```python
from build123d import *

# Parameters (mm, degrees)
SKETCH1_R              = 9.525
BOSS_EXTRUDE1_DEPTH    = 3
CUT_EXTRUDE1_DEPTH     = 72.404901793
SKETCH4_W              = 50.8
SKETCH4_H              = 19.4
BOSS_EXTRUDE3_DEPTH    = 6
SKETCH3_W              = 6
SKETCH3_H              = 12.7
BOSS_EXTRUDE2_DEPTH    = 6
FILLET1_R              = 1.5875
LPATTERN1_COUNT        = 5
LPATTERN1_PITCH        = 25.4
FILLET1_OF_LPATTERN1_R = 1.5875
SKETCH5_W              = 12.7
SKETCH5_H              = 6
BOSS_EXTRUDE4_DEPTH    = 6
FILLET2_R              = 1.5875
LPATTERN2_COUNT        = 2
LPATTERN2_PITCH        = 25.4
FILLET2_OF_LPATTERN2_R = 1.5875


with BuildPart() as part:
    # Sketch1 → Boss-Extrude1 (new, symmetric)
    with BuildSketch(Plane(origin=(0, 0, 0), x_dir=(0, 0, -1), z_dir=(1, 0, 0))):
        with BuildLine():
            Line((-15.540953853, 3.23950279), (-9.525, 32.1))
            Line((-9.525, 32.1), (63.5, 32.1))
            Line((63.5, 32.1), (63.5, -15.875))
            Line((63.5, -15.875), (0, -15.875))
            ThreePointArc((0, -15.875), (-12.317522717, -10.014702148), (-15.540953853, 3.23950279))
        make_face()
        Circle(SKETCH1_R, mode=Mode.SUBTRACT)
    extrude(amount=BOSS_EXTRUDE1_DEPTH, both=True)

    # Sketch2 → Cut-Extrude1 (cut, through all)
    with BuildSketch(Plane(origin=(3, 0, 0), x_dir=(0, 0, -1), z_dir=(1, 0, 0))):
        with BuildLine():
            Line((1.676231888, -15.786255783), (23.396510982, -13.47993154))
            ThreePointArc((23.396510982, -13.47993154), (24.056064004, -13.361605673), (24.691925535, -13.150202478))
            Line((24.691925535, -13.150202478), (53.43843719, -1.24300748))
            ThreePointArc((53.43843719, -1.24300748), (54.045535898, -0.938110333), (54.602034594, -0.548443406))
            Line((54.602034594, -0.548443406), (63.5, 6.7))
            Line((63.5, 6.7), (63.5, -15.875))
            Line((63.5, -15.875), (0, -15.875))
            ThreePointArc((0, -15.875), (0.839289711, -15.852798421), (1.676231888, -15.786255783))
        make_face()
        with BuildLine():
            Line((26.903135362, 18.016834009), (41.56972294, 24.091933498))
            ThreePointArc((41.56972294, 24.091933498), (49.866397767, 20.655338262), (46.429802531, 12.358663435))
            Line((46.429802531, 12.358663435), (31.763214953, 6.283563946))
            ThreePointArc((31.763214953, 6.283563946), (23.466540126, 9.720159182), (26.903135362, 18.016834009))
        make_face()
        with BuildLine():
            Line((22.328855341, -7.445246365), (51.075366995, 4.461948633))
            ThreePointArc((51.075366995, 4.461948633), (53.035211442, 3.650154483), (52.223417292, 1.690310036))
            Line((52.223417292, 1.690310036), (23.476905638, -10.216884962))
            ThreePointArc((23.476905638, -10.216884962), (21.51706119, -9.405090812), (22.328855341, -7.445246365))
        make_face()
        with BuildLine():
            Line((12.055034553, 17.357951117), (40.801546208, 29.265146115))
            ThreePointArc((40.801546208, 29.265146115), (42.761390655, 28.453351965), (41.949596505, 26.493507518))
            Line((41.949596505, 26.493507518), (13.203084851, 14.58631252))
            ThreePointArc((13.203084851, 14.58631252), (11.243240403, 15.39810667), (12.055034553, 17.357951117))
        make_face()
    extrude(amount=-CUT_EXTRUDE1_DEPTH, mode=Mode.SUBTRACT)

    # Sketch4 → Boss-Extrude3 (add)
    with BuildSketch(Plane(origin=(3, 0, 0), x_dir=(0, 0, -1), z_dir=(1, 0, 0))):
        with Locations((88.9, 22.4)):
            Rectangle(SKETCH4_W, SKETCH4_H)
    extrude(amount=-BOSS_EXTRUDE3_DEPTH)

    # Sketch3 → Boss-Extrude2 (add)
    with BuildSketch(Plane(origin=(0, 32.1, 0), x_dir=(1, 0, 0), z_dir=(0, 1, 0))):
        Rectangle(SKETCH3_W, SKETCH3_H)
    boss_extrude2 = extrude(amount=BOSS_EXTRUDE2_DEPTH)

    # Fillet1
    fillet1_edges = [part.edges().sort_by_distance(p)[0] for p in [
        (0, 38.1, -6.35),
        (0, 38.1, 6.35),
    ]]
    fillet(fillet1_edges, radius=FILLET1_R)

    # LPattern1: Boss-Extrude2 ×5
    with Locations(*[(0, 0, -i * LPATTERN1_PITCH) for i in range(1, LPATTERN1_COUNT)]):
        add(boss_extrude2)

    # Fillet1 of LPattern1
    fillet1_of_lpattern1_edges = [part.edges().sort_by_distance(p)[0] for p in [
        (0, 38.1, -31.75),
        (0, 38.1, -19.05),
        (0, 38.1, -57.15),
        (0, 38.1, -44.45),
        (0, 38.1, -82.55),
        (0, 38.1, -69.85),
        (0, 38.1, -107.95),
        (0, 38.1, -95.25),
    ]]
    fillet(fillet1_of_lpattern1_edges, radius=FILLET1_OF_LPATTERN1_R)

    # Sketch5 → Boss-Extrude4 (add)
    with BuildSketch(Plane.ZY.offset(3)):
        with Locations((-76.2, 9.7)):
            Rectangle(SKETCH5_W, SKETCH5_H)
    boss_extrude4 = extrude(amount=-BOSS_EXTRUDE4_DEPTH)

    # Fillet2
    fillet2_edges = [part.edges().sort_by_distance(p)[0] for p in [
        (0, 6.7, -82.55),
        (0, 6.7, -69.85),
    ]]
    fillet(fillet2_edges, radius=FILLET2_R)

    # LPattern2: Boss-Extrude4 ×2
    with Locations(*[(0, 0, -i * LPATTERN2_PITCH) for i in range(1, LPATTERN2_COUNT)]):
        add(boss_extrude4)

    # Fillet2 of LPattern2
    fillet2_of_lpattern2_edges = [part.edges().sort_by_distance(p)[0] for p in [
        (0, 6.7, -107.95),
        (0, 6.7, -95.25),
    ]]
    fillet(fillet2_of_lpattern2_edges, radius=FILLET2_OF_LPATTERN2_R)


solid = part.part
```
Geometry check sheet. Reference: the model listing, model coordinates, mm. A direction names the side the tool comes from. Give positions to 0.01 mm unless a question says otherwise; leave off trailing zeros. Write each loop counter-clockwise with the first axis right and the second up, starting at its lowest first coordinate (ties: lowest second). Pieces come first, ordered by that corner, then holes. Notation, with made-up numbers: (-19.5, -38.5) - (29.5, -38.5) arc R21 cw to (29.5, -16.5) - close; hole circle Ø5 at (78, 4). An arc over 180 degrees is marked (long way). Use a Markdown table: item, result.
Q1. Thickness scan on L1, parallel to Y at x = 0.9, z = 0 (3 decimals); L2, parallel to Z at x = 1.75, y = -6.5; L3, parallel to Z at x = 1.75, y = 23. Record the ranges inside material, lowest first. Write a range as [from, to].
Computed:
| item | result |
|---|---|
| L1 | y = [-15.875, -9.525], [9.525, 38.1] |
| L2 | z = [-40.75, -32.45], [-24.61, -6.96], [6.96, 14.48] |
| L3 | z = [-114.3, -48.19], [-38.93, -33.52], [-25.68, 11.42] |
Q2. Section check B-B, the plane z = -35.5. Enter the section's corners in (x, y), then the cut area to 3 significant figures.
Computed:
| item | result |
|---|---|
| outline | (-3, -8.67) - (3, -8.67) - (3, -5.24) - (-3, -5.24) - close; (-3, -1.99) - (3, -1.99) - (3, 7.83) - (-3, 7.83) - close; (-3, 21.58) - (3, 21.58) - (3, 23.82) - (-3, 23.82) - close; (-3, 27.07) - (3, 27.07) - (3, 32.1) - (-3, 32.1) - close |
| area | 123 mm² |
Q3. Section check A-A, the plane y = -3. Enter the section's corners in (x, z).
Computed:
| item | result |
|---|---|
| outline | (-3, -49.2) - (3, -49.2) - (3, -40.9) - (-3, -40.9) - close; (-3, -33.06) - (3, -33.06) - (3, -9.04) - (-3, -9.04) - close; (-3, 9.04) - (3, 9.04) - (3, 15.59) - (-3, 15.59) - close |
Q4. Go/stop test with flat-tipped pins: P1, Ø1.5, axis at x = 2, y = -7, coming from the -Z side; P2, Ø3, axis at x = -0.5, z = -39.5, coming from the +Y side; P3, Ø2, axis at x = 1.5, y = 34, coming from the +Z side; P4, Ø5, axis at y = 4, z = -79, coming from the +X side. Record where each tip stops, or that it passes through.
Computed:
| item | result |
|---|---|
| P1 | stops at z = -41.35 |
| P2 | stops at y = 32.1 |
| P3 | stops at z = 6.35 |
| P4 | passes through |
Q5. Set-up check for faces 5 (the face through (0, 12.7, -67)), 6 (the face through (0, 34, 6.35)), 7 (the face through (0, 34, -69.85)): record each of +Z, -Z, +X, -X, +Y, -Y from which the full face is reachable in a straight line by a thin tool's end or side.
Computed:
| item | result |
|---|---|
| face 5 | +X, -X, -Y |
| face 6 | +Z, +X, -X, +Y |
| face 7 | +X, -X, +Y |
Q6. Draft check along Y on faces 1 (the face through (0, 34, -107.95)), 2 (the face through (0.042, 3.68, -53.022)), 3 (the face through (0.042, -1.575, -36.501)), 4 (the face through (0, 38.1, 0)). Enter one of: pulls with the +Y half, pulls with the -Y half, needs draft (parallel to the pull), parting line crosses it, or undercut.
Computed:
| item | result |
|---|---|
| face 1 | needs draft |
| face 2 | undercut |
| face 3 | undercut |
| face 4 | pulls with the +Y half |
Q7. Section check C-C, the plane x = -1. Give the number of separate pieces and of enclosed holes in the cut face, then the cut area to 3 significant figures.
Computed:
| item | result |
|---|---|
| separate pieces | 1 |
| enclosed holes | 4 |
| area | 3,890 mm² |
